For this review, take the finished solid that the model builds, in its own axes (mm). Face numbers are marked on the shaded views. A direction names the side the tool comes from. Give positions to 0.01 mm unless a question says otherwise; leave off trailing zeros. Order: outer loops, then holes, each group sorted by start corner. A loop starts at its lowest first (then second) coordinate and runs counter-clockwise, first axis right, second up. Notation, with made-up numbers: (4.5, -25.75) -> (32.5, -25.75) arc R17 cw to (32.5, -16.75) -> close; hole circle Ø6 at (2.25, 89.25). An arc over 180 degrees is marked (long way). Return JSON: item names as keys, results as strings. Group by question number.
1) To check wall thickness, follow line 1 along Z through (x, y) = (-17.5, 14.5) (3 decimals); line 2 along Y through (x, z) = (23.5, 41.5); line 3 along Y through (x, z) = (31, 43). State the ranges of each line that lie inside material, in increasing order.
2) Insertion check: P1, Ø12, axis at x = 48, z = 23, coming from the +Y side; P2, Ø14, axis at y = 17, z = 21.5, coming from the -X side (3 decimals); P3, Ø16.5, axis at x = 0, y = -31, coming from the +Z side (3 decimals); P4, Ø12, axis at x = 56, y = 25.5, coming from the +Z side (3 decimals). Each pin has a flat end and moves straight along its axis. Give the tip position at first contact, or say it passes through.
3) Add section B-B (z = -3). Give the boundary of the cut face in (x, y) (3 decimals).
4) For the marked faces 4, 5, 6 and 7, list the 3-axis set-ups (+Z, -Z, +X, -X, +Y, -Y) from which the entire face can be reached by the end or side of a thin tool; tool diameter is ignored.
5) Add section A-A (x = 95). Give the boundary of the cut face in (y, z) (3 decimals), then the cut area to 3 significant figures.
6) The part is to be moulded in two halves that separate along X. For the marked faces 1, 2 and 3, say which applies: released by +X, released by -X, zero draft, split by the parting line, or undercut.
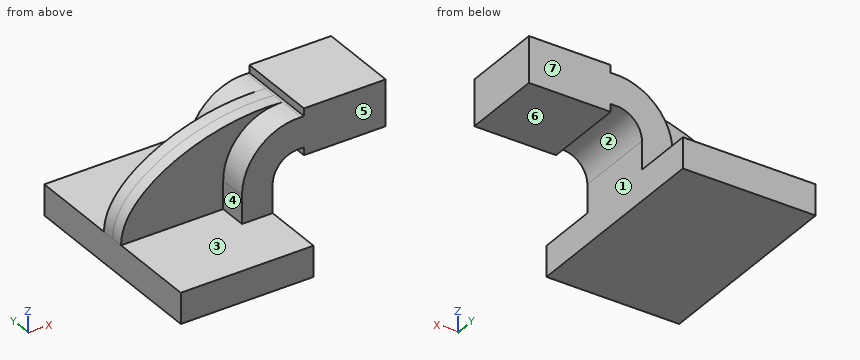
from build123d import *

# Parameters (mm, degrees)
F1_DEPTH = 63.5
F2_DEPTH = 25.4
F3_DEPTH = 7.9375


with BuildPart() as f1:
    # F0 (on Front) → F1 (new body, symmetric)
    with BuildSketch(Plane.XZ):
        Polygon((41.275, -9.525), (41.275, 9.525), (22.225, 9.525), (-41.275, 9.525), (-41.275, -9.525), align=None)
    extrude(amount=F1_DEPTH, both=True)

    # F0 (on Front) → F2 (join, symmetric)
    with BuildSketch(Plane.XZ):
        with BuildLine():
            Line((22.225, 9.525), (41.275, 9.525))
            Line((41.275, 9.525), (41.275, 27.055227))
            ThreePointArc((41.275, 27.055227), (46.40173, 38.738134), (58.470631, 42.8752))
            Line((58.470631, 42.8752), (60.744337, 42.8752))
            Line((60.744337, 42.8752), (60.744337, 61.9252))
            Line((60.744337, 61.9252), (59.109739, 61.9252))
            ThreePointArc((59.109739, 61.9252), (33.15717, 52.434347), (22.225, 27.055227))
            Line((22.225, 27.055227), (22.225, 9.525))
        make_face()
        Polygon((60.744337, 61.9252), (60.744337, 42.8752), (60.744337, 38.1), (111.544337, 38.1), (111.544337, 66.675), (60.744337, 66.675), align=None)
    extrude(amount=F2_DEPTH, both=True)

    # F0 (on Front) → F3 (join, symmetric)
    with BuildSketch(Plane.XZ):
        Polygon((60.744337, 61.9252), (60.744337, 42.8752), (60.744337, 38.1), (111.544337, 38.1), (111.544337, 66.675), (60.744337, 66.675), align=None)
        Polygon((41.275, -9.525), (41.275, 9.525), (22.225, 9.525), (-41.275, 9.525), (-41.275, -9.525), align=None)
        with BuildLine():
            Line((22.225, 9.525), (41.275, 9.525))
            Line((41.275, 9.525), (41.275, 27.055227))
            ThreePointArc((41.275, 27.055227), (46.40173, 38.738134), (58.470631, 42.8752))
            Line((58.470631, 42.8752), (60.744337, 42.8752))
            Line((60.744337, 42.8752), (60.744337, 61.9252))
            Line((60.744337, 61.9252), (59.109739, 61.9252))
            ThreePointArc((59.109739, 61.9252), (33.15717, 52.434347), (22.225, 27.055227))
            Line((22.225, 27.055227), (22.225, 9.525))
        make_face()
        with BuildLine():
            Line((-41.275, 9.525), (22.225, 9.525))
            Line((22.225, 9.525), (22.225, 27.055227))
            ThreePointArc((22.225, 27.055227), (33.15717, 52.434347), (59.109739, 61.9252))
            add(Edge.make_bspline(
                [(-41.275, 9.525), (-41.747715, 40.443104), (11.415395, 65.556966), (59.109739, 61.9252)],
                knots=[0, 0, 0, 0, 113.238142, 113.238142, 113.238142, 113.238142], degree=3))
        make_face()
    extrude(amount=F3_DEPTH, both=True)


solid = f1.part
Evaluation:
{
 "1": {"line 1": "-9.525 to 9.525", "line 2": "-7.94 to 7.94", "line 3": "-25.4 to 25.4"},
 "2": {"P1": "through", "P2": "x = 22.225", "P3": "z = 9.525", "P4": "z = 66.675"},
 "3": {"outline": "(-41.275, -63.5) -> (41.275, -63.5) -> (41.275, 63.5) -> (-41.275, 63.5) -> close"},
 "4": {"face 4": "+Z, -X, -Y", "face 5": "+Z, +X, -X, -Y", "face 6": "-Z, +X, +Y, -Y", "face 7": "+Z, +X, -X, +Y"},
 "5": {"outline": "(-25.4, 38.1) -> (25.4, 38.1) -> (25.4, 66.675) -> (-25.4, 66.675) -> close", "area": "1,450 mm^2"},
 "6": {"face 1": "released by +X", "face 2": "undercut", "face 3": "zero draft"}
}
